Check sheet for the modelled part. Datum: model origin and axes. Units: mm. Face numbers are marked on the shaded views. A direction names the side the tool comes from. Round coordinates to 2 decimals unless told otherwise and drop trailing zeros. Write each loop counter-clockwise with the first axis right and the second up, starting at its lowest first coordinate (ties: lowest second). Pieces come first, ordered by that corner, then holes. Notation, with made-up numbers: (-22, 18) -> (-17, 18) arc R33 ccw to (-17, 54) -> close; hole circle Ø9 at (-38, 63). An arc over 180 degrees is marked (long way). One line per item, written item: value.
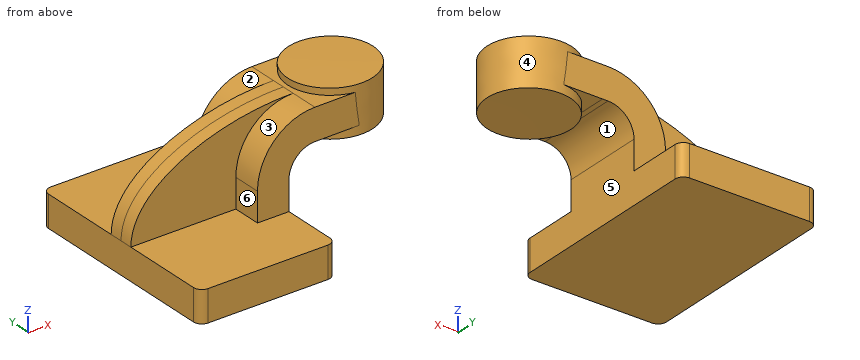
from build123d import *

# Parameters (mm, degrees)
F1_DEPTH = 63.5
F2_DEPTH = 25.4
F3_DEPTH = 7.9375
F5_R     = 5.08


with BuildPart() as f1:
    # F0 (on Front) → F1 (new body, symmetric)
    with BuildSketch(Plane.XZ):
        Polygon((22.225, 9.525), (-41.275, 9.525), (-41.275, -9.525), (41.275, -9.525), (41.275, 9.525), align=None)
    extrude(amount=F1_DEPTH, both=True)

    # F0 (on Front) → F2 (join, symmetric)
    with BuildSketch(Plane.XZ):
        with BuildLine():
            Line((22.225, 27.1089508341), (22.225, 9.525))
            Line((22.225, 9.525), (41.275, 9.525))
            Line((41.275, 9.525), (41.275, 27.1089508341))
            ThreePointArc((41.275, 27.1089508341), (45.8865944339, 38.2960559133), (57.0420954398, 42.9835841088))
            Line((57.0420954398, 42.9835841088), (60.325, 43.0058989785))
            Line((60.325, 43.0058989785), (60.325, 62.056339059))
            Line((60.325, 62.056339059), (56.9126099675, 62.0331440384))
            ThreePointArc((56.9126099675, 62.0331440384), (32.3705077545, 51.7205820083), (22.225, 27.1089508341))
        make_face()
        Polygon((85.3500794925, 62.2264418986), (60.325, 62.056339059), (60.325, 43.0058989785), (85.4795649648, 43.176881969), (85.3787372937, 61.4743826337), align=None)
    extrude(amount=F2_DEPTH, both=True)

    # F0 (on Front) → F3 (join, symmetric)
    with BuildSketch(Plane.XZ):
        with BuildLine():
            add(Edge.make_bspline(
                [(-41.275, 9.525), (-41.1433540285, 41.4384305477), (10.1432753727, 62.2998327017), (56.9126099675, 62.0331440384)],
                knots=[0, 0, 0, 0, 111.3459112023, 111.3459112023, 111.3459112023, 111.3459112023], degree=3))
            Line((-41.275, 9.525), (22.225, 9.525))
            Line((22.225, 9.525), (22.225, 27.1089508341))
            ThreePointArc((22.225, 27.1089508341), (32.3705077545, 51.7205820083), (56.9126099675, 62.0331440384))
        make_face()
    extrude(amount=F3_DEPTH, both=True)

    # F0 (on Front) → F4 (revolve)
    with BuildSketch(Plane.XZ):
        Polygon((111.125, 66.675), (85.3500794925, 66.675), (85.4390979857, 59.8903526073), (85.725, 38.1), (111.125, 38.1), align=None)
    revolve(axis=Axis((85.5375397462, 0, 52.3875), (0.0131194485, 0, -0.9999139363)))

    # F5
    f5_edges = [f1.edges().sort_by_distance(p)[0] for p in [
        (41.275, -63.5, 0),
        (-41.275, -63.5, 0),
        (-41.275, 63.5, 0),
        (41.275, 63.5, 0),
    ]]
    fillet(f5_edges, radius=F5_R)


solid = f1.part
Item 1: Depth check by flat-ended pin: P1, Ø2, axis at x = 29.5, z = 17.5, coming from the +Y side; P2, Ø12, axis at x = 81, y = 27, coming from the -Z side; P3, Ø8, axis at y = 25, z = 29, coming from the -X side (3 decimals). Enter the tip coordinate at first touch or a pass-through.
Answer:
P1: stops at y = 25.4
P2: stops at z = 37.64
P3: stops at x = 22.225
Item 2: Thickness scan on line 1 (X direction, y = -8.5, z = 13.5) (3 decimals); line 2 (X direction, y = -58, z = -0.5) (3 decimals); line 3 (Z direction, x = -33.5, y = -41) (3 decimals). Record the ranges inside material, lowest first.
Answer:
line 1: x = 22.225 to 41.275
line 2: x = -41.275 to 41.275
line 3: z = -9.525 to 9.525
Item 3: Sectioned sample at B-B on y = -45. Enter the section's corners in (x, z) (3 decimals), and give its area (3 significant figures).
Answer:
outline: (-41.275, -9.525) -> (41.275, -9.525) -> (41.275, 9.525) -> (-41.275, 9.525) -> close
area: 1,570 mm^2
Item 4: Sectioned sample at A-A on z = -5. Enter the section's corners in (x, y) (3 decimals), and give its area (3 significant figures).
Answer:
outline: (-41.275, -58.42) arc R5.08 ccw to (-36.195, -63.5) -> (36.195, -63.5) arc R5.08 ccw to (41.275, -58.42) -> (41.275, 58.42) arc R5.08 ccw to (36.195, 63.5) -> (-36.195, 63.5) arc R5.08 ccw to (-41.275, 58.42) -> close
area: 10,500 mm^2
Item 5: Tool access check on the marked faces 1, 2 and 3. Record the directions out of +Z, -Z, +X, -X, +Y, -Y that give a thin tool (end or side, any length) a straight path to the whole face; none if there is none.
Answer:
face 1: -Z, +Y, -Y
face 2: +Z, -X, +Y
face 3: +Z, -X, -Y
Item 6: Mould release check, pull along X, two halves, no side actions. Record for the marked faces 4, 5 and 6: pulls with the +X half, pulls with the -X half, needs draft (parallel to the pull), parting line crosses it, or undercut.
Answer:
face 4: undercut
face 5: pulls with the +X half
face 6: pulls with the -X half
